Check sheet for the modelled part. Datum: model origin and axes. Units: mm. Face numbers are marked on the shaded views. A direction names the side the tool comes from. Coordinates: 2 decimals unless noted, no trailing zeros. Loops run counter-clockwise (first coordinate to the right, second up) from the corner with the lowest first, then second, coordinate; pieces in that order, holes last. Notation, with made-up numbers: (68, 80) -> (110, 80) arc R17 cw to (110, 90) -> close; hole circle Ø7 at (43.5, 35.25). An arc over 180 degrees is marked (long way). Use CSV: the item, a comma, the result in double quotes.
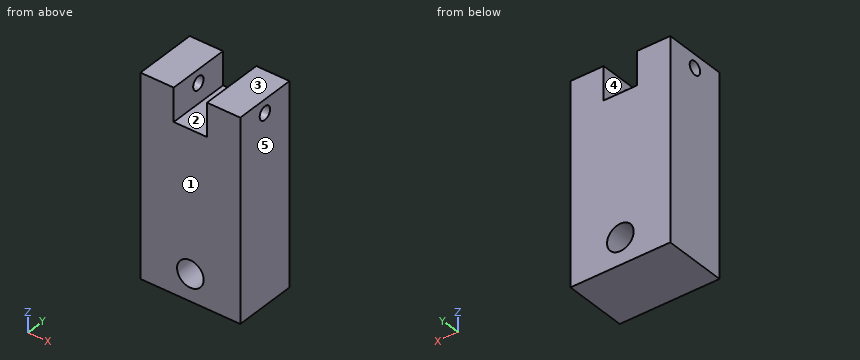
```python
from build123d import *

# Parameters (mm, degrees)
BOSS_EXTRUDE1_DEPTH = 95
SKETCH3_R           = 20
CUT_EXTRUDE2_DEPTH  = 327
SKETCH4_R           = 10
CUT_EXTRUDE3_DEPTH  = 260
SKETCH5_W           = 50
SKETCH5_H           = 95.125248012
CUT_EXTRUDE4_DEPTH  = 50
SCALE1_SCALE        = 0.75


with BuildPart() as part:
    # Sketch1 → Boss-Extrude1 (new body)
    with BuildSketch(Plane(origin=(0, 0, 0), x_dir=(1, 0, 0), z_dir=(0, 1, 0))):
        Polygon((72.999601763, 104.000796475), (97.999601763, 104.000796475), (97.999601763, -195.999203525), (72.999601763, -195.999203525), (22.999601763, -195.999203525), (-52.000398237, -195.999203525), (-52.000398237, 104.000796475), (22.999601763, 104.000796475), align=None)
    extrude(amount=BOSS_EXTRUDE1_DEPTH)

    # Sketch3 → Cut-Extrude2 (cut)
    with BuildSketch(Plane(origin=(0, 95, 0), x_dir=(1, 0, 0), z_dir=(0, 1, 0))):
        with Locations(Location((22.999601763, 64.000796475, 0), (0, 0, 270))):
            Circle(SKETCH3_R)
    extrude(amount=-CUT_EXTRUDE2_DEPTH, mode=Mode.SUBTRACT)

    # Sketch4 → Cut-Extrude3 (cut)
    with BuildSketch(Plane(origin=(97.999601763, 0, 0), x_dir=(0, 0, -1), z_dir=(1, 0, 0))):
        with Locations((-175.999203525, 47.5)):
            Circle(SKETCH4_R)
    extrude(amount=-CUT_EXTRUDE3_DEPTH, mode=Mode.SUBTRACT)

    # Sketch5 → Cut-Extrude4 (cut)
    with BuildSketch(Plane.XY.offset(195.999203525)):
        with Locations((22.999601763, 47.562624006)):
            Rectangle(SKETCH5_W, SKETCH5_H)
    extrude(amount=-CUT_EXTRUDE4_DEPTH, mode=Mode.SUBTRACT)


with BuildPart() as part_1:
    # Scale1: scaled about (22.999601763, 47.5, 40.688864602)
    add(part.part.scale(SCALE1_SCALE).moved(Location((5.749900441, 11.875, 10.172216151))))


solid = part_1.part
```
1) Draft check along X on the marked faces 3, 4 and 5. Enter one of: released by +X, released by -X, zero draft, split by the parting line, or undercut.
Answer below:
face 3,"zero draft"
face 4,"undercut"
face 5,"released by +X"
2) Thickness scan on line 1 along Z through (x, y) = (-4, 47); line 2 along X through (y, z) = (73.5, 145.5); line 3 along Z through (x, y) = (11, 36.5). Record the ranges inside material, lowest first. Write a range as from..to.
Answer below:
line 1,"z = -67.83..134.69, 149.65..157.17"
line 2,"x = -33.25..4.25, 41.75..79.25"
line 3,"z = -67.83..-46.83, -28.83..119.67"
3) Access from +Z, -Z, +X, -X, +Y, -Y to the whole of each face (thin tool, end or side, straight path). Record for the marked faces 1 and 2.
Answer below:
face 1,"+Z, -Z, +X, -X, -Y"
face 2,"+Z, +Y, -Y"
4) Cross-section at B-B on y = 68. Record the boundary of the cut face in (x, z), and give its area (3 significant figures).
Answer below:
outline,"(-33.25, -67.83) -> (79.25, -67.83) -> (79.25, 157.17) -> (41.75, 157.17) -> (41.75, 119.67) -> (4.25, 119.67) -> (4.25, 157.17) -> (-33.25, 157.17) -> close; hole circle Ø30 at (23, -37.83)"
area,"23,200 mm²"
5) Cross-section at A-A on y = 47.5. Record the boundary of the cut face in (x, z), and give its area (3 significant figures).
Answer below:
outline,"(-33.25, -67.83) -> (79.25, -67.83) -> (79.25, 134.67) -> (41.75, 134.67) -> (41.75, 119.67) -> (4.25, 119.67) -> (4.25, 134.67) -> (-33.25, 134.67) -> close; (-33.25, 149.67) -> (4.25, 149.67) -> (4.25, 157.17) -> (-33.25, 157.17) -> close; (41.75, 149.67) -> (79.25, 149.67) -> (79.25, 157.17) -> (41.75, 157.17) -> close; hole circle Ø30 at (23, -37.83)"
area,"22,100 mm²"
6) Go/stop test with a flat-tipped pin: pin 1 Ø2 at (x, y) = (14, 58) entering from +Z. Record where the tip stops, or that it passes through.
Answer below:
pin 1,"stops at z = 119.67"
